Geometry check sheet. Reference: the model listing, model coordinates, mm. A direction names the side the tool comes from. Give positions to 0.01 mm unless a question says otherwise; leave off trailing zeros. Write each loop counter-clockwise with the first axis right and the second up, starting at its lowest first coordinate (ties: lowest second). Pieces come first, ordered by that corner, then holes. Notation, with made-up numbers: M -27,82 L 5,82 A23 ccw 5,94 Z; hole C 56.25,-16 d3. An arc over 180 degrees is marked long. Use one line per item in the form item = value. Start each with the question number.
Solid Edge part; units mm, degrees
sketch "Sketch1" plane through (0, 0, 0) normal (0, 0, 1) x (1, 0, 0)
  circle A0 centre (-59.1628, -18.1899) radius 1
  line L0 (-40.0782, -20.6709) -> (-40.0782, -36.2909)
  arc A1 (-40.0782, -36.2909) -> (-41.0782, -37.2909) centre (-41.0782, -36.2909) cw
  line L1 (-41.0782, -37.2909) -> (-56.6982, -37.2909)
  line L2 (-60.5782, -33.4109) -> (-56.6982, -37.2909)
  line L3 (-60.5782, -33.4109) -> (-60.5782, -17.9909)
  arc A2 (-60.5782, -17.9909) -> (-59.3782, -16.7909) centre (-59.3782, -17.9909) cw
  line L4 (-59.3782, -16.7909) -> (-43.9582, -16.7909)
  line L5 (-43.9582, -16.7909) -> (-40.0782, -20.6709)
  circle A3 centre (-41.4332, -35.9309) radius 1
extrude "Protrusion1" add sketch "Sketch1" along normal blind 4.7
sketch "Sketch2" plane through (-50.3282, -27.0409, 4.7) normal (0, 0, 1) x (0, -1, 0)
  circle A0 centre (0, 0) radius 4.25
  arc A1 (-10.25, -3.9922) -> (-3.9922, -10.25) centre (0, 0) ccw
  line L0 (-3.9922, -10.25) -> (3.9922, -10.25)
  arc A2 (3.9922, -10.25) -> (10.25, -3.9922) centre (0, 0) ccw
  line L1 (10.25, 3.9922) -> (10.25, -3.9922)
  arc A3 (3.9922, 10.25) -> (10.25, 3.9922) centre (0, 0) cw
  line L2 (-3.9922, 10.25) -> (3.9922, 10.25)
  arc A4 (-3.9922, 10.25) -> (-10.25, 3.9922) centre (0, 0) ccw
  line L3 (-10.25, 3.9922) -> (-10.25, -3.9922)
extrude "ExtrudedProtrusion_2" add sketch "Sketch2" along normal blind 1.1
sketch "Sketch3" plane through (-50.3282, -27.0409, 5.8) normal (0, 0, 1) x (1, 0, 0)
  circle A0 centre (0, 0) radius 7
extrude "ExtrudedProtrusion_3" add sketch "Sketch3" along normal blind 1
sketch "Sketch4" plane through (-50.3282, -27.0409, 6.8) normal (0, 0, 1) x (1, 0, 0)
  circle A0 centre (0, 0) radius 2
extrude "ExtrudedProtrusion_4" add sketch "Sketch4" along normal blind 1.5
sketch "Sketch5" plane through (-50.3282, -27.0409, 8.3) normal (0, 0, 1) x (1, 0, 0)
  circle A0 centre (0, 0) radius 10
extrude "ExtrudedProtrusion_5" add sketch "Sketch5" along normal blind 2
sketch "Sketch6" plane through (-50.3282, 0, 0) normal (1, 0, 0) x (0, 1, 0)
  line L0 (-37.0409, 9.1255) -> (-37.0409, 10.3)
  line L1 (-37.0409, 10.3) -> (-27.0409, 10.3)
  line L2 (-27.0409, 10.3) -> (-27.0409, 4.8545)
  arc A0 (-27.0409, 9.3) -> (-35.898, 10.0828) centre (-27.0409, 59.8) cw
  arc A1 (-35.898, 10.0828) -> (-37.0409, 9.1255) centre (-36.0685, 9.1255) ccw
revolve "RevolvedCutout1" cut sketch "Sketch6" angle 360 about axis through (-50.3282, -27.0409, 10.3) along (0, 0, -1)
sketch "Sketch7" plane through (-48.8882, -37.2909, 2.9) normal (0, -1, 0) x (1, 0, 0)
  line L0 (-6.69, -0.7104) -> (-6.69, -2.7104)
  line L1 (-6.69, -2.7104) -> (3.81, -2.7104)
  line L2 (3.81, -2.7104) -> (3.81, -0.7104)
  line L3 (3.81, -0.7104) -> (-6.69, -0.7104)
extrude "ExtrudedProtrusion_6" add sketch "Sketch7" along normal blind 4
(1) Sectioned sample at A-A, the plane z = 4. Record the boundary of the cut face in (x, y).
(2) Tool access check on faces 4 (the cylindrical face through (-58.264, -20.956, 8.707)), 5 (the cylindrical face through (-42.595, -19.218, 5.242)), 6 (the flat face through (-55.578, -39, 1)), 7 (the cylindrical face through (-58.151, -19.308, 5.242)), 8 (the flat face through (-50, -27, 4.7)). Record the directions out of +Z, -Z, +X, -X, +Y, -Y that give a thin tool (end or side, any length) a straight path to the whole face; none if there is none.
(3) Sectioned sample at D-D, the plane z = 5.5. Record the boundary of the cut face in (x, y).
(4) Draft check along Y on faces 1 (the cylindrical face through (-58.625, -19.033, 2.317)), 2 (the flat face through (-42.05, -18.7, 2.32)), 3 (the cylindrical face through (-40.363, -36.99, 2.317)). Enter one of: released by +Y, released by -Y, zero draft, split by the parting line, or undercut.
(5) Sectioned sample at B-B, the plane x = -53.25. State how many separate pieces and enclosed holes the cut face has, plus the area to 3 significant figures.
(6) Thickness scan on probe 1 along Z at (x, y) = (-48.5, -28); probe 2 along Z at (x, y) = (-47, -38.5); probe 3 along Y at (x, z) = (-52.25, 2.5). Record the ranges inside material, lowest first. Write a range as [from, to].
(7) Depth check by flat-ended pin: pin 1 (2.5 mm diameter, centred on x = -41.43, y = -35.93, fed in from +Z); pin 2 (2 mm diameter, centred on y = -39, z = 1, fed in from +X); pin 3 (2.5 mm diameter, centred on x = -51.5, y = -26, fed in from +Z). Enter the tip coordinate at first touch or a pass-through.
Numbers:
q1.outline = M -60.58,-33.41 L -56.7,-37.29 L -41.08,-37.29 A1 ccw -40.08,-36.29 L -40.08,-20.67 L -43.96,-16.79 L -59.38,-16.79 A1.2 ccw -60.58,-17.99 Z; hole C -59.16,-18.19 d2; hole C -41.43,-35.93 d2
q2.face_4 = +Z
q2.face_5 = +Z, +X, +Y
q2.face_6 = +Z, -Z, -X, -Y
q2.face_7 = +Z, -X, +Y
q2.face_8 = none
q3.outline = M -60.58,-31.03 A11 ccw -54.32,-37.29 L -46.34,-37.29 A11 ccw -40.08,-31.03 L -40.08,-23.05 A11 ccw -46.34,-16.79 L -54.32,-16.79 A11 ccw -60.58,-23.05 Z; hole C -50.33,-27.04 d8.5
q4.face_1 = undercut
q4.face_2 = released by +Y
q4.face_3 = released by -Y
q5.separate_pieces = 2
q5.enclosed_holes = 1
q5.area = 159 mm2
q6.probe_1 = [0, 4.7], [5.8, 6.8], [8.3, 9.34]
q6.probe_2 = [0.19, 2.19]
q6.probe_3 = [-37.29, -16.79]
q7.pin_1 = 4.7
q7.pin_2 = -45.08
q7.pin_3 = 9.38
